Design review of the part built by this model. Coordinates are the model's own, in mm. A direction names the side the tool comes from. Give positions to 0.01 mm unless a question says otherwise; leave off trailing zeros. Order: outer loops, then holes, each group sorted by start corner. A loop starts at its lowest first (then second) coordinate and runs counter-clockwise, first axis right, second up.
```python
from build123d import *

# Parameters (mm, degrees)
BOSS_EXTRUDE1_DEPTH = 4


with BuildPart() as part:
    # Sketch1 → Boss-Extrude1 (new body)
    with BuildSketch(Plane.XY):
        with BuildLine():
            Line((0, 0), (10, 0))
            Line((10, 0), (10, -4))
            Line((10, -4), (20, -4))
            Line((20, -4), (20, 0))
            Line((20, 0), (30, 0))
            Line((30, 0), (30, -4))
            Line((30, -4), (40, -4))
            Line((40, -4), (40, 0))
            Line((40, 0), (50, 0))
            Line((50, 0), (50, 10))
            ThreePointArc((50, 10), (25, 52.632453378), (0, 10))
            Line((0, 10), (0, 0))
        make_face()
    extrude(amount=BOSS_EXTRUDE1_DEPTH)


solid = part.part
```
1. For pin 1 (2 mm diameter, centred on y = -1.5, z = 2, fed in from +X); pin 2 (2 mm diameter, centred on y = -2.5, z = 3, fed in from -X); pin 3 (2 mm diameter, centred on x = 5, z = 1.5, fed in from -Y), all flat-tipped, find the tip position at first contact; note any pin that passes through.
Recorded:
pin 1: stops at x = 40
pin 2: stops at x = 10
pin 3: stops at y = 0
2. Take a section at C-C (x = 25). State the section outline as (y, z) points, then the cut area to 3 significant figures.
Recorded:
outline: (0, 0) - (52.63, 0) - (52.63, 4) - (0, 4) - close
area: 211 mm2
3. For line 1 along X through (y, z) = (8.5, 1.65); line 2 along X through (y, z) = (10.5, 1.2); line 3 along Y through (x, z) = (39, 2.2), list the stretches that pass through material, from the lowest coordinate up.
Recorded:
line 1: x = 0 to 50
line 2: x = -0.27 to 50.27
line 3: y = -4 to 48.98
4. Take a section at B-B (y = 6). State the section outline as (x, z) points, then the cut area to 3 significant figures.
Recorded:
outline: (0, 0) - (50, 0) - (50, 4) - (0, 4) - close
area: 200 mm2
5. Machinability: for faces 5 (the face through (15, -4, 2)), 6 (the face through (20, -2, 2)), 7 (the face through (25.83, 52.62, 1.97)), 8 (the face through (10, -2, 2)), 9 (the face through (45, 0, 2)), which of the approach directions +Z, -Z, +X, -X, +Y, -Y give a long, thin tool a straight path to every point of the face, cutting with its end or side? Answer none if there is none.
Recorded:
face 5: +Z, -Z, +X, -X, -Y
face 6: +Z, -Z, -Y
face 7: +Z, -Z
face 8: +Z, -Z, -X, -Y
face 9: +Z, -Z, +X, -Y
6. Draft analysis for pull direction X (two halves, no side actions). For faces 1 (the face through (50, 5, 2)), 2 (the face through (30, -2, 2)), 3 (the face through (25, 0, 2)), 4 (the face through (5, 0, 2)), state which applies: pulls with the +X half, pulls with the -X half, needs draft (parallel to the pull), parting line crosses it, or undercut.
Recorded:
face 1: pulls with the +X half
face 2: undercut
face 3: undercut
face 4: needs draft
7. Take a section at A-A (z = 2.15). State the section outline as (x, y) points, then the cut area to 3 significant figures.
Recorded:
outline: (0, 0) - (10, 0) - (10, -4) - (20, -4) - (20, 0) - (30, 0) - (30, -4) - (40, -4) - (40, 0) - (50, 0) - (50, 10) arc R28.65 ccw (long way) to (0, 10) - close
area: 2,640 mm2
